from build123d import *

# Parameters (mm, degrees)
SKETCH_1_R      = 12
SKETCH_1_R_2    = 1
SKETCH_1_R_3    = 1.5
EXTRUDE_1_DEPTH = 3
SKETCH_2_R      = 4
SKETCH_2_R_2    = 1.5
EXTRUDE_2_DEPTH = 3


with BuildPart() as part:
    # 草图1 → 凸台-拉伸1 (new body)
    with BuildSketch(Plane.XY):
        Circle(SKETCH_1_R)
        with Locations((0, 8)):
            Circle(SKETCH_1_R_2, mode=Mode.SUBTRACT)
        with Locations((5.656854249, 5.656854249)):
            Circle(SKETCH_1_R_2, mode=Mode.SUBTRACT)
        with Locations((8, 0)):
            Circle(SKETCH_1_R_2, mode=Mode.SUBTRACT)
        with Locations((5.656854249, -5.656854249)):
            Circle(SKETCH_1_R_2, mode=Mode.SUBTRACT)
        with Locations((0, -8)):
            Circle(SKETCH_1_R_2, mode=Mode.SUBTRACT)
        with Locations((-5.656854249, -5.656854249)):
            Circle(SKETCH_1_R_2, mode=Mode.SUBTRACT)
        with Locations((-8, 0)):
            Circle(SKETCH_1_R_2, mode=Mode.SUBTRACT)
        with Locations((-5.656854249, 5.656854249)):
            Circle(SKETCH_1_R_2, mode=Mode.SUBTRACT)
        Circle(SKETCH_1_R_3, mode=Mode.SUBTRACT)
    extrude(amount=EXTRUDE_1_DEPTH)

    # 草图2 → 凸台-拉伸2 (add)
    with BuildSketch(Plane.XY.offset(3)):
        Circle(SKETCH_2_R)
        Circle(SKETCH_2_R_2, mode=Mode.SUBTRACT)
    extrude(amount=EXTRUDE_2_DEPTH)


solid = part.part
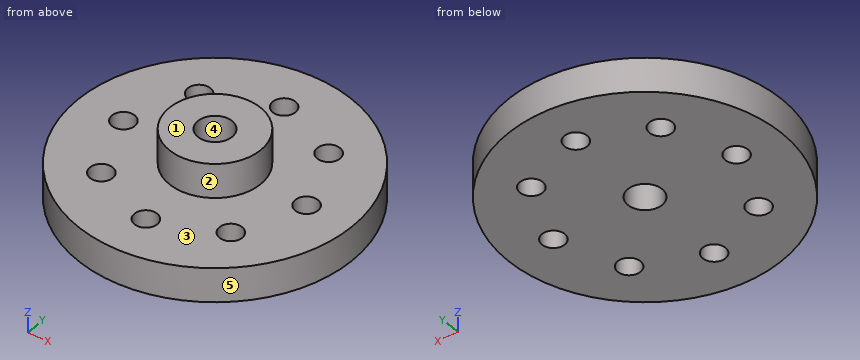
The model under review builds one solid part; all positions refer to its coordinate system, in mm. Face numbers are marked on the shaded views. A direction names the side the tool comes from. Coordinates: 2 decimals unless noted, no trailing zeros. Loops run counter-clockwise (first coordinate to the right, second up) from the corner with the lowest first, then second, coordinate; pieces in that order, holes last.
(1) Wall thickness on L1, parallel to Y at x = 0, z = 0.95; L2, parallel to Z at x = 7.75, y = 4; L3, parallel to X at y = 1.25, z = 2.7: over which ranges is each line inside the solid? List them lowest first.
Determined:
L1: y = -12 to -9, -7 to -1.5, 1.5 to 7, 9 to 12
L2: z = 0 to 3
L3: x = -11.93 to -0.83, 0.83 to 11.93
(2) Consider section A-A, the plane x = 0. Give the boundary of the cut face in (y, z).
Determined:
outline: (-12, 0) - (-9, 0) - (-9, 3) - (-12, 3) - close; (-7, 0) - (-1.5, 0) - (-1.5, 6) - (-4, 6) - (-4, 3) - (-7, 3) - close; (1.5, 0) - (7, 0) - (7, 3) - (4, 3) - (4, 6) - (1.5, 6) - close; (9, 0) - (12, 0) - (12, 3) - (9, 3) - close
(3) Tool access review of the marked faces 1 and 2: name each direction out of +Z, -Z, +X, -X, +Y, -Y from which nothing blocks a thin tool from reaching the whole face with its end or side.
Determined:
face 1: +Z, +X, -X, +Y, -Y
face 2: +Z
(4) Consider section C-C, the plane z = 4.9. Give the boundary of the cut face in (x, y), plus the area to 3 significant figures.
Determined:
outline: circle Ø8 at (0, 0); hole circle Ø3 at (0, 0)
area: 43.2 mm2
(5) Insertion check: P1, Ø7, axis at x = -5, y = -3.5, coming from the +Z side; P2, Ø2.5, axis at x = 5.66, y = -5.66, coming from the +Z side; P3, Ø1.5, axis at x = 4, z = 2.5, coming from the -Y side; P4, Ø3, axis at y = 9, z = 3.5, coming from the -X side. Each pin has a flat end and moves straight along its axis. Give the tip position at first contact, or say it passes through.
Determined:
P1: stops at z = 6
P2: stops at z = 3
P3: stops at y = -11.55
P4: stops at x = -9.3
(6) Consider section B-B, the plane x = 8. Give the boundary of the cut face in (y, z), plus the area to 3 significant figures.
Determined:
outline: (-8.94, 0) - (-1, 0) - (-1, 3) - (-8.94, 3) - close; (1, 0) - (8.94, 0) - (8.94, 3) - (1, 3) - close
area: 47.7 mm2
(7) Draft analysis for pull direction X (two halves, no side actions). For the marked faces 3, 4 and 5, state which applies: +X half, -X half, draft (parallel to the pull), parting line (faces both ways), or undercut.
Determined:
face 3: draft
face 4: undercut
face 5: parting line
